from build123d import *

# Parameters (mm, degrees)
F0_W     = 76.2
F0_H     = 50.8
F0_R     = 12.7
F1_DEPTH = 6.35
F2_W     = 6.35
F2_H     = 50.8
F3_DEPTH = 2.54
F5_DEPTH = 25.4
F6_R     = 2.54
F7_DEPTH = 12.7


# Not quite as in the source:
# - a feature names something its author has since deleted; it is built from what else it names


with BuildPart() as f1:
    # F0 (on Top) → F1 (new body)
    with BuildSketch(Plane.XY):
        Rectangle(F0_W, F0_H)
        Circle(F0_R, mode=Mode.SUBTRACT)
    extrude(amount=-F1_DEPTH)

    # F2 (on face) → F3 (cut)
    with BuildSketch(Plane.XY):
        with Locations((-32.385, 0)):
            Rectangle(F2_W, F2_H)
        with BuildLine():
            Line((-5.08, -11.6397422652), (-5.08, -25.4))
            Line((-5.08, -25.4), (5.08, -25.4))
            Line((5.08, -25.4), (5.08, -11.6397422652))
            ThreePointArc((5.08, -11.6397422652), (0, -12.7), (-5.08, -11.6397422652))
        make_face()
        with BuildLine():
            Line((5.08, 25.4), (-5.08, 25.4))
            Line((-5.08, 25.4), (-5.08, 11.6397422652))
            ThreePointArc((-5.08, 11.6397422652), (0, 12.7), (5.08, 11.6397422652))
            Line((5.08, 11.6397422652), (5.08, 25.4))
        make_face()
    extrude(amount=-F3_DEPTH, mode=Mode.SUBTRACT)

    # F4 (on Front) → F5 (cut, symmetric)
    with BuildSketch(Plane.XZ):
        Polygon((31.75, 0), (19.05, 0), (16.1170606325, -5.08), (34.6859807152, -5.08), align=None)
    extrude(amount=F5_DEPTH, both=True, mode=Mode.SUBTRACT)

    # F6 (on face) → F7 (join)
    with BuildSketch(Plane.YZ.offset(38.1)):
        with Locations((0, -3.81)):
            Circle(F6_R)
    extrude(amount=F7_DEPTH)


solid = f1.part
The model under review builds one solid part; all positions refer to its coordinate system, in mm. A direction names the side the tool comes from. Round coordinates to 2 decimals unless told otherwise and drop trailing zeros. Loops run counter-clockwise (first coordinate to the right, second up) from the corner with the lowest first, then second, coordinate; pieces in that order, holes last. Notation, with made-up numbers: (86, 82.5) -> (121, 82.5) arc R16 cw to (121, 92.5) -> close; hole circle Ø1 at (28, -17). An arc over 180 degrees is marked (long way). Write item = value, one per line. Start each with the question number.
Item 1: Mouldability with a two-part tool opening along Y and no side actions: class faces 1 (the cylindrical face through (12.114, 3.815, -3.131)), 2 (the flat face through (8, 12, -6.35)), 3 (the flat face through (-1, -25.4, -3)) as released by +Y, released by -Y, zero draft, split by the parting line, or undercut.
Item 2: To check wall thickness, follow L1, parallel to Y at x = 0, z = -3.75; L2, parallel to X at y = 11.5, z = -0.5; L3, parallel to X at y = 8, z = -4.75. State the ranges of each line that lie inside material, in increasing order.
Item 3: Take a section at A-A on x = 0. Give the boundary of the cut face in (y, z), plus the area to 3 significant figures.
Item 4: For faces 4 (the flat face through (-35.56, 0, -1)), 5 (the cylindrical face through (44.361, 2.423, -3.047)), 6 (the flat face through (17.604, -0.356, -2.504)), list the 3-axis set-ups (+Z, -Z, +X, -X, +Y, -Y) from which the entire face can be reached by the end or side of a thin tool; tool diameter is ignored.
Item 5: Take a section at B-B on y = -19. Give the boundary of the cut face in (x, z).
Item 6: Take a section at C-C on z = -3.81. Give the boundary of the cut face in (x, y).
Item 7: Insertion check: pin 1 (2 mm diameter, centred on y = -9, z = -0.5, fed in from +X); pin 2 (3 mm diameter, centred on x = -0.5, y = 19.5, fed in from +Z). Each pin has a flat end and moves straight along its axis. Give the tip position at first contact, or say it passes through.
Item 8: Take a section at D-D on y = -6. Give the boundary of the cut face in (x, z), plus the area to 3 significant figures.
Result:
q1.face_1 = undercut
q1.face_2 = zero draft
q1.face_3 = released by -Y
q2.L1 = -25.4 to -12.7, 12.7 to 25.4
q2.L2 = -38.1 to -35.56, -29.21 to -5.39, 5.39 to 18.76, 32.04 to 38.1
q2.L3 = -38.1 to -9.86, 9.86 to 16.31, 34.5 to 38.1
q3.outline = (-25.4, -6.35) -> (-12.7, -6.35) -> (-12.7, -2.54) -> (-25.4, -2.54) -> close; (12.7, -6.35) -> (25.4, -6.35) -> (25.4, -2.54) -> (12.7, -2.54) -> close
q3.area = 96.8 mm²
q4.face_4 = +Z, +Y, -Y
q4.face_5 = +X
q4.face_6 = +Y, -Y
q5.outline = (-38.1, -6.35) -> (38.1, -6.35) -> (38.1, 0) -> (31.75, 0) -> (34.69, -5.08) -> (16.12, -5.08) -> (19.05, 0) -> (5.08, 0) -> (5.08, -2.54) -> (-5.08, -2.54) -> (-5.08, 0) -> (-29.21, 0) -> (-29.21, -2.54) -> (-35.56, -2.54) -> (-35.56, 0) -> (-38.1, 0) -> close
q6.outline = (-38.1, -25.4) -> (16.85, -25.4) -> (16.85, 25.4) -> (-38.1, 25.4) -> close; (33.95, -25.4) -> (38.1, -25.4) -> (38.1, -2.54) -> (50.8, -2.54) -> (50.8, 2.54) -> (38.1, 2.54) -> (38.1, 25.4) -> (33.95, 25.4) -> close; hole circle Ø25.4 at (0, 0)
q7.pin_1 = 38.1
q7.pin_2 = -2.54
q8.outline = (-38.1, -6.35) -> (-11.19, -6.35) -> (-11.19, 0) -> (-29.21, 0) -> (-29.21, -2.54) -> (-35.56, -2.54) -> (-35.56, 0) -> (-38.1, 0) -> close; (11.19, -6.35) -> (38.1, -6.35) -> (38.1, 0) -> (31.75, 0) -> (34.69, -5.08) -> (16.12, -5.08) -> (19.05, 0) -> (11.19, 0) -> close
q8.area = 246 mm²
